Check sheet for the modelled part. Datum: model origin and axes. Units: mm. A direction names the side the tool comes from. Coordinates: 2 decimals unless noted, no trailing zeros. Order: outer loops, then holes, each group sorted by start corner. A loop starts at its lowest first (then second) coordinate and runs counter-clockwise, first axis right, second up. Notation, with made-up numbers: (6, -35) -> (29, -35) arc R28 cw to (29, 2) -> close; hole circle Ø11 at (-17.75, -13). An arc over 180 degrees is marked (long way). Put each result on its own line as item: value. Start each with the question number.
```python
from build123d import *

# Parameters (mm, degrees)
F1_DEPTH = 1.5


# Not quite as in the source:
# - ends of sketch curves that miss each other by under 0.0002 mm in the source are joined


with BuildPart() as f1:
    # F0 (on Top) → F1 (new body)
    with BuildSketch(Plane.XY):
        Polygon((-34.6231374532, -30.5467036664), (-34.6231374532, -35.0467036664), (-31.8731374532, -35.0467036664), (-30.6230945961, -35.0467036664), (-26.6231374532, -35.0467036664), (-26.6231374532, -30.5467036664), (-30.6230517389, -30.5467036664), align=None)
        with BuildLine():
            Line((-30.6230945961, -35.0467036664), (-31.8731374532, -35.0467036664))
            ThreePointArc((-31.8731374532, -35.0467036664), (-31.1952175422, -35.1833094776), (-30.6231474562, -35.5718611088))
            Line((-30.6231474562, -35.5718611088), (-30.6230945961, -35.0467036664))
        make_face()
        with BuildLine():
            Line((-26.6231374532, -35.0467036664), (-30.6230945961, -35.0467036664))
            Line((-30.6230945961, -35.0467036664), (-30.6231474562, -35.5718611088))
            ThreePointArc((-30.6231474562, -35.5718611088), (-30.1230517371, -36.796737), (-30.6231941178, -38.0215938389))
            Line((-30.6231941178, -38.0215938389), (-30.6232041199, -38.5467036666))
            Line((-30.6232041199, -38.5467036666), (-26.6232041199, -38.5467036666))
            Line((-26.6232041199, -38.5467036666), (-26.6231374532, -35.0467036664))
        make_face()
        with BuildLine():
            ThreePointArc((-30.6231941178, -38.0215938389), (-30.1230517371, -36.796737), (-30.6231474562, -35.5718611088))
            Line((-30.6231474562, -35.5718611088), (-30.6231941178, -38.0215938389))
        make_face()
        with BuildLine():
            Line((-30.6232041199, -38.5467036666), (-30.6231941178, -38.0215938389))
            ThreePointArc((-30.6231941178, -38.0215938389), (-31.1951692504, -38.410077566), (-31.8729660246, -38.5467036666))
            Line((-31.8729660246, -38.5467036666), (-30.6232041199, -38.5467036666))
        make_face()
        Polygon((-26.6234136437, -49.5467036666), (-26.6232041199, -38.5467036666), (-30.6232041199, -38.5467036666), (-30.6234136437, -49.5467036665), align=None)
        Polygon((-30.6234136437, -49.5467036665), (-30.6232041199, -38.5467036666), (-31.8729660246, -38.5467036666), (-34.6229279294, -38.5467036666), (-34.6231374532, -49.5467036664), (-31.8734136439, -49.5467036665), align=None)
        with BuildLine():
            Line((-26.6234803104, -53.0467036664), (-26.6234136437, -49.5467036666))
            Line((-26.6234136437, -49.5467036666), (-30.6234136437, -49.5467036665))
            Line((-30.6234136437, -49.5467036665), (-30.623423649, -50.0719826043))
            ThreePointArc((-30.623423649, -50.0719826043), (-30.1234469771, -51.2967369998), (-30.6234703059, -52.5214723478))
            Line((-30.6234703059, -52.5214723478), (-30.6234803104, -53.0467036664))
            Line((-30.6234803104, -53.0467036664), (-26.6234803104, -53.0467036664))
        make_face()
        with BuildLine():
            Line((-30.623423649, -50.0719826043), (-30.6234136437, -49.5467036665))
            Line((-30.6234136437, -49.5467036665), (-31.8734136439, -49.5467036665))
            ThreePointArc((-31.8734136439, -49.5467036665), (-31.1954794965, -49.6833654824), (-30.623423649, -50.0719826043))
        make_face()
        Polygon((-26.6235660246, -57.5467036664), (-26.6234803104, -53.0467036664), (-30.6234803104, -53.0467036664), (-31.8734803104, -53.0467036664), (-34.6234803104, -53.0467036664), (-34.6234803104, -57.5467036664), align=None)
        with BuildLine():
            ThreePointArc((-30.6234703059, -52.5214723478), (-30.1234469771, -51.2967369998), (-30.623423649, -50.0719826043))
            Line((-30.623423649, -50.0719826043), (-30.6234703059, -52.5214723478))
        make_face()
        with BuildLine():
            Line((-31.8734803104, -53.0467036664), (-30.6234803104, -53.0467036664))
            Line((-30.6234803104, -53.0467036664), (-30.6234703059, -52.5214723478))
            ThreePointArc((-30.6234703059, -52.5214723478), (-31.1955409574, -52.9100676767), (-31.8734803104, -53.0467036665))
        make_face()
    extrude(amount=F1_DEPTH)


solid = f1.part
```
1) Sectioned sample at B-B (z = 0.95). Record the boundary of the cut face in (x, y), plus the area to 3 significant figures.
2) Scan lines: line 1 along Y through (x, z) = (-33.75, 1.3); line 2 along Y through (x, z) = (-30.75, 0.8); line 3 along X through (y, z) = (-52, 0.2). Record each from-to range of solid material in increasing order. Write a range as [from, to].
3) Mould release check, pull along Y, two halves, no side actions. Record for faces 3 (the flat face through (-33, -38.547, 1)), 4 (the flat face through (-31, -44, 1.5)), 5 (the flat face through (-31, -57.547, 1)): +Y half, -Y half, draft (parallel to the pull), parting line (faces both ways), or undercut.
4) Sectioned sample at C-C (x = -31.25). Record the boundary of the cut face in (y, z).
5) Sectioned sample at A-A (x = -33.75). Record the boundary of the cut face in (y, z).
6) Sectioned sample at D-D (y = -36). Record the boundary of the cut face in (x, z).
7) Access from +Z, -Z, +X, -X, +Y, -Y to the whole of each face (thin tool, end or side, straight path). Record for faces 1 (the cylindrical face through (-31.2, -35.18, 0.74)), 2 (the flat face through (-34.623, -55, 1)).
Entries:
1. outline: (-34.62, -57.55) -> (-26.62, -57.55) -> (-26.62, -35.05) -> (-26.62, -30.55) -> (-34.62, -30.55) -> (-34.62, -35.05) -> (-31.87, -35.05) arc R1.75 cw to (-30.62, -35.57) -> (-30.62, -38.02) arc R1.75 cw to (-31.87, -38.55) -> (-34.62, -38.55) -> (-34.62, -49.55) -> (-31.87, -49.55) arc R1.75 cw to (-30.62, -50.07) -> (-30.62, -52.52) arc R1.75 cw to (-31.87, -53.05) -> (-34.62, -53.05) -> close
1. area: 189 mm2
2. line 1: y = [-57.55, -53.05], [-49.55, -38.55], [-35.05, -30.55]
2. line 2: y = [-57.55, -52.64], [-49.95, -38.14], [-35.45, -30.55]
2. line 3: x = [-30.62, -26.62]
3. face 3: undercut
3. face 4: draft
3. face 5: -Y half
4. outline: (-57.55, 0) -> (-52.93, 0) -> (-52.93, 1.5) -> (-57.55, 1.5) -> close; (-49.66, 0) -> (-38.43, 0) -> (-38.43, 1.5) -> (-49.66, 1.5) -> close; (-35.16, 0) -> (-30.55, 0) -> (-30.55, 1.5) -> (-35.16, 1.5) -> close
5. outline: (-57.55, 0) -> (-53.05, 0) -> (-53.05, 1.5) -> (-57.55, 1.5) -> close; (-49.55, 0) -> (-38.55, 0) -> (-38.55, 1.5) -> (-49.55, 1.5) -> close; (-35.05, 0) -> (-30.55, 0) -> (-30.55, 1.5) -> (-35.05, 1.5) -> close
6. outline: (-30.62, 0) -> (-26.62, 0) -> (-26.62, 1.5) -> (-30.62, 1.5) -> close
7. face 1: +Z, -Z, -X
7. face 2: +Z, -Z, -X, +Y, -Y
